Could you check a few things on this model? Use its own coordinates, in mm. Coordinates: 2 decimals unless noted, no trailing zeros. Loops run counter-clockwise (first coordinate to the right, second up) from the corner with the lowest first, then second, coordinate; pieces in that order, holes last.
1) Imagine slicing it at B-B on z = 312.5. Please give me the cut outline in (x, y), plus the area to 3 significant figures.
2) Imagine slicing it at C-C on x = 163. Please give me the cut outline in (y, z).
3) If I drill on line 1 along X through (y, z) = (-1.75, -265); line 2 along Z through (x, y) = (179, -4.45); line 3 along Z through (x, y) = (-349, -0.3), over which ranges is the centre line in solid material (lowest first)?
4) Imagine slicing it at A-A on y = -1.2. Please give me the cut outline in (x, z), plus the area to 3 significant figures.
5) Will these pins go through, and if not, where does the flat tip stop? P1, Ø3, axis at y = -1, z = -344.5, coming from the +X side; P2, Ø2, axis at y = -5.5, z = 339, coming from the +X side.
```python
from build123d import *

# Parameters (mm, degrees)
F1_DEPTH = 6


with BuildPart() as f1:
    # F0 (on Front) → F1 (new body)
    with BuildSketch(Plane.XZ):
        with BuildLine():
            Line((-415, 600), (-572, 600))
            Line((-572, 600), (-572, -262))
            Line((-572, -262), (-381, -262))
            ThreePointArc((-381, -262), (-355, -236), (-329, -262))
            Line((-329, -262), (-301, -262))
            ThreePointArc((-301, -262), (-275, -236), (-249, -262))
            ThreePointArc((-249, -262), (-256.6152236891, -280.3847763109), (-275, -288))
            Line((-275, -288), (-275, -597))
            Line((-275, -597), (575, -597))
            Line((575, -597), (575, -410))
            Line((575, -410), (-415, 600))
        make_face()
        with BuildLine():
            Line((-381, -262), (-572, -262))
            Line((-572, -262), (-572, -597))
            Line((-572, -597), (-355, -597))
            Line((-355, -597), (-355, -288))
            ThreePointArc((-355, -288), (-373.3847763109, -280.3847763109), (-381, -262))
        make_face()
        with BuildLine():
            Line((-301, -262), (-329, -262))
            ThreePointArc((-329, -262), (-336.6152236891, -280.3847763109), (-355, -288))
            Line((-355, -288), (-355, -597))
            Line((-355, -597), (-275, -597))
            Line((-275, -597), (-275, -288))
            ThreePointArc((-275, -288), (-293.3847763109, -280.3847763109), (-301, -262))
        make_face()
    extrude(amount=F1_DEPTH)


solid = f1.part
```
Filled in:
1. outline: (-572, -6) - (-133.19, -6) - (-133.19, 0) - (-572, 0) - close
1. area: 2,630 mm2
2. outline: (-6, -597) - (0, -597) - (0, 10.32) - (-6, 10.32) - close
3. line 1: x = -572 to -380.83, -329.17 to -300.83, -249.17 to 432.87
3. line 2: z = -597 to -6
3. line 3: z = -597 to -287.3, -236.7 to 532.67
4. outline: (-572, -597) - (575, -597) - (575, -410) - (-415, 600) - (-572, 600) - close; hole circle Ø52 at (-355, -262); hole circle Ø52 at (-275, -262)
4. area: 869,000 mm2
5. P1: stops at x = 512.27
5. P2: stops at x = -158.19
